Part model, mm, in its own coordinate system. A direction names the side the tool comes from. Give positions to 0.01 mm unless a question says otherwise; leave off trailing zeros. Write each loop counter-clockwise with the first axis right and the second up, starting at its lowest first coordinate (ties: lowest second). Pieces come first, ordered by that corner, then holes.
```python
from build123d import *

# Parameters (mm, degrees)
SKETCH1_W           = 5.58
SKETCH1_H           = 4.83
BOSS_EXTRUDE1_DEPTH = 6.345
SKETCH2_W           = 1.19
SKETCH2_H           = 1.68
BOSS_EXTRUDE2_DEPTH = 2.09
SKETCH4_W           = 3.2
SKETCH4_H           = 0.4
BOSS_EXTRUDE3_DEPTH = 2.09


with BuildPart() as part:
    # Sketch1 → Boss-Extrude1 (new, symmetric)
    with BuildSketch(Plane(origin=(0, 0, 0), x_dir=(1, 0, 0), z_dir=(0, 1, 0))):
        Rectangle(SKETCH1_W, SKETCH1_H)
    extrude(amount=BOSS_EXTRUDE1_DEPTH, both=True)

    # Sketch2 → Boss-Extrude2 (add)
    with BuildSketch(Plane(origin=(0, 6.345, 0), x_dir=(1, 0, 0), z_dir=(0, 1, 0))):
        with Locations((-2.195, 3.255)):
            Rectangle(SKETCH2_W, SKETCH2_H)
        with Locations((2.195, 3.255)):
            Rectangle(SKETCH2_W, SKETCH2_H)
    extrude(amount=-BOSS_EXTRUDE2_DEPTH)

    # Sketch4 → Boss-Extrude3 (add)
    with BuildSketch(Plane(origin=(0, 6.345, 0), x_dir=(1, 0, 0), z_dir=(0, 1, 0))):
        with Locations((0, 2.615)):
            Rectangle(SKETCH4_W, SKETCH4_H)
    extrude(amount=-BOSS_EXTRUDE3_DEPTH)


solid = part.part
```
1) Pin check, flat tips, straight feed: pin 1 Ø1.3 at (x, z) = (0.5, -3.5) entering from -Y; pin 2 Ø1 at (x, y) = (0, 5.5) entering from -Z (3 decimals); pin 3 Ø1 at (x, y) = (-0.5, 2.5) entering from -Z (3 decimals). Stop position of each tip, or through.
Answers follow:
pin 1: passes through
pin 2: stops at z = -2.815
pin 3: stops at z = -2.415
2) Saw through at C-C, the plane x = 0.1. Write the cut outline in (y, z) (3 decimals).
Answers follow:
outline: (-6.345, -2.415) - (4.255, -2.415) - (4.255, -2.815) - (6.345, -2.815) - (6.345, 2.415) - (-6.345, 2.415) - close
3) 3-axis set-ups, long thin cutter, end or side, ignore diameter. For faces 1 (the face through (0, 6.345, -1)), 2 (the face through (-1.6, 5, -3)), 3 (the face through (0, -1, -2.415)): which of +Z, -Z, +X, -X, +Y, -Y reach the whole face in a straight line?
Answers follow:
face 1: +Z, -Z, +X, -X, +Y
face 2: -Z, +Y, -Y
face 3: -Z, +X, -X, -Y
4) Saw through at A-A, the plane z = -3. Write the cut outline in (x, y) (3 decimals), then the cut area to 3 significant figures.
Answers follow:
outline: (-2.79, 4.255) - (-1.6, 4.255) - (-1.6, 6.345) - (-2.79, 6.345) - close; (1.6, 4.255) - (2.79, 4.255) - (2.79, 6.345) - (1.6, 6.345) - close
area: 4.97 mm2
5) Wall check: L1, parallel to X at y = 5.75, z = -3; L2, parallel to Z at x = 0.4, y = 3 (3 decimals); L3, parallel to Y at x = 1.8, z = -3.5 (3 decimals). Give the ranges that are in metal, low to high.
Answers follow:
L1: x = -2.79 to -1.6, 1.6 to 2.79
L2: z = -2.415 to 2.415
L3: y = 4.255 to 6.345
6) Saw through at B-B, the plane y = 4.75. Write the cut outline in (x, z) (3 decimals).
Answers follow:
outline: (-2.79, -4.095) - (-1.6, -4.095) - (-1.6, -2.815) - (1.6, -2.815) - (1.6, -4.095) - (2.79, -4.095) - (2.79, 2.415) - (-2.79, 2.415) - close
7) Saw through at D-D, the plane y = -3.25. Write the cut outline in (x, z) (3 decimals).
Answers follow:
outline: (-2.79, -2.415) - (2.79, -2.415) - (2.79, 2.415) - (-2.79, 2.415) - close
8) Two-plate mould, pull along X, no slides. Class faces 4 (the face through (-2, 5, -4.095)), 5 (the face through (0, 5, -2.815)), 6 (the face through (-2.79, 0, 0)): +X half, -X half, draft (parallel to the pull), parting line (faces both ways), or undercut.
Answers follow:
face 4: draft
face 5: undercut
face 6: -X half
